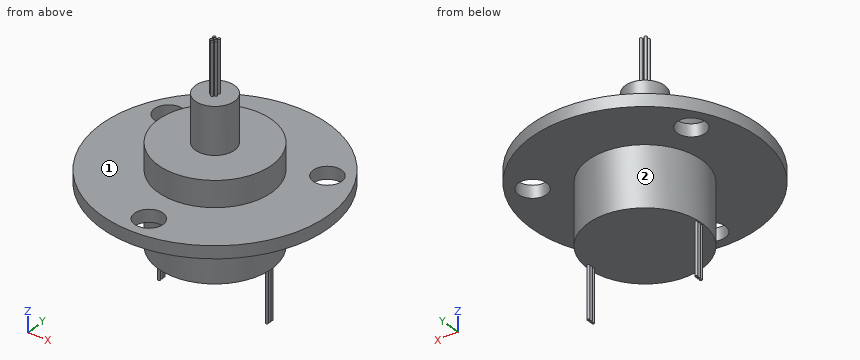
```python
from build123d import *

# Parameters (mm, degrees)
SKETCH1_W                      = 22
SKETCH1_H                      = 2.4
SKETCH2_R                      = 11
BOSS_EXTRUDE1_DEPTH            = 5
SKETCH3_R                      = 3.8
BOSS_EXTRUDE2_DEPTH            = 9
SKETCH4_R                      = 0.25
BOSS_EXTRUDE3_DEPTH            = 10
SKETCH5_R                      = 11
BOSS_EXTRUDE4_DEPTH            = 11.6
SKETCH6_W                      = 0.25
SKETCH6_H                      = 10
SKETCH7_W                      = 0.25
SKETCH7_H                      = 10
SKETCH8_W                      = 0.25
SKETCH8_H                      = 10
SKETCH9_W                      = 0.25
SKETCH9_H                      = 10
SKETCH10_W                     = 0.25
SKETCH10_H                     = 10
SKETCH11_W                     = 0.25
SKETCH11_H                     = 10
SKETCH12_W                     = 0.25
SKETCH12_H                     = 10
SKETCH13_W                     = 0.25
SKETCH13_H                     = 10
SKETCH14_W                     = 0.25
SKETCH14_H                     = 10
SKETCH15_W                     = 0.25
SKETCH15_H                     = 10
SKETCH16_W                     = 0.25
SKETCH16_H                     = 10
F_5_5_5_5_DIAMETER_HOLE1_D     = 5.5
F_5_5_5_5_DIAMETER_HOLE1_DEPTH = 26.4


with BuildPart() as part:
    # Sketch1 → Revolve1 (revolve)
    with BuildSketch(Plane.XZ):
        with Locations((11, 1.2)):
            Rectangle(SKETCH1_W, SKETCH1_H)
    revolve(axis=Axis((0, 0, 2.4), (0, 0, -1)))

    # Sketch2 → Boss-Extrude1 (add)
    with BuildSketch(Plane.XY.offset(2.4)):
        Circle(SKETCH2_R)
    extrude(amount=BOSS_EXTRUDE1_DEPTH)

    # Sketch3 → Boss-Extrude2 (add)
    with BuildSketch(Plane.XY.offset(7.4)):
        Circle(SKETCH3_R)
    extrude(amount=BOSS_EXTRUDE2_DEPTH)

    # Sketch4 → Boss-Extrude3 (add)
    with BuildSketch(Plane.XY.offset(16.4)):
        Circle(SKETCH4_R)
    extrude(amount=BOSS_EXTRUDE3_DEPTH)

    # Sketch5 → Boss-Extrude4 (add)
    with BuildSketch(Plane(origin=(0, 0, 0), x_dir=(-1, 0, 0), z_dir=(0, 0, -1))):
        Circle(SKETCH5_R)
    extrude(amount=BOSS_EXTRUDE4_DEPTH)

    # Sketch6 → Revolve2 (revolve)
    with BuildSketch(Plane.XZ.offset(0.816347149)):
        with Locations((0.163253006, 21.4)):
            Rectangle(SKETCH6_W, SKETCH6_H)
    revolve(axis=Axis((0.038253006, -0.816347149, 26.4), (0, 0, -1)))

    # Sketch7 → Revolve3 (revolve)
    with BuildSketch(Plane.XZ.offset(0.416347149)):
        with Locations((0.613253006, 21.4)):
            Rectangle(SKETCH7_W, SKETCH7_H)
    revolve(axis=Axis((0.488253006, -0.416347149, 26.4), (0, 0, -1)))

    # Sketch8 → Revolve4 (revolve)
    with BuildSketch(Plane.XZ.offset(-0.383652851)):
        with Locations((-0.286746994, 21.4)):
            Rectangle(SKETCH8_W, SKETCH8_H)
    revolve(axis=Axis((-0.411746994, 0.383652851, 26.4), (0, 0, -1)))

    # Sketch9 → Revolve5 (revolve)
    with BuildSketch(Plane.XZ.offset(-0.400094572)):
        with Locations((0.572352369, 21.4)):
            Rectangle(SKETCH9_W, SKETCH9_H)
    revolve(axis=Axis((0.447352369, 0.400094572, 26.4), (0, 0, -1)))

    # Sketch10 → Revolve6 (revolve)
    with BuildSketch(Plane(origin=(0, -0.222432877, 0), x_dir=(1, 0, 0), z_dir=(0, 1, 0))):
        with Locations((-10.392433295, 16.6)):
            Rectangle(SKETCH10_W, SKETCH10_H)
    revolve(axis=Axis((-10.517433295, -0.222432877, -21.6), (0, 0, 1)))

    # Sketch11 → Revolve7 (revolve)
    with BuildSketch(Plane(origin=(0, 0.377567123, 0), x_dir=(1, 0, 0), z_dir=(0, 1, 0))):
        with Locations((-10.392433295, 16.6)):
            Rectangle(SKETCH11_W, SKETCH11_H)
    revolve(axis=Axis((-10.517433295, 0.377567123, -21.6), (0, 0, 1)))

    # Sketch12 → Revolve8 (revolve)
    with BuildSketch(Plane(origin=(0, 0.6, 0), x_dir=(1, 0, 0), z_dir=(0, 1, 0))):
        with Locations((10.496693215, 16.6)):
            Rectangle(SKETCH12_W, SKETCH12_H)
    revolve(axis=Axis((10.371693215, 0.6, -21.6), (0, 0, 1)))

    # Sketch13 → Revolve9 (revolve)
    with BuildSketch(Plane(origin=(0, 0, 0), x_dir=(1, 0, 0), z_dir=(0, 1, 0))):
        with Locations((10.496693215, 16.6)):
            Rectangle(SKETCH13_W, SKETCH13_H)
    revolve(axis=Axis((10.371693215, 0, -21.6), (0, 0, 1)))

    # Sketch14 → Revolve10 (revolve)
    with BuildSketch(Plane(origin=(0, -0.6, 0), x_dir=(1, 0, 0), z_dir=(0, 1, 0))):
        with Locations((10.496693215, 16.6)):
            Rectangle(SKETCH14_W, SKETCH14_H)
    revolve(axis=Axis((10.371693215, -0.6, -21.6), (0, 0, 1)))

    # Sketch15 → Revolve11 (revolve)
    with BuildSketch(Plane(origin=(0, 0.968647222, 0), x_dir=(1, 0, 0), z_dir=(0, 1, 0))):
        with Locations((-10.392433295, 16.6)):
            Rectangle(SKETCH15_W, SKETCH15_H)
    revolve(axis=Axis((-10.517433295, 0.968647222, -21.6), (0, 0, 1)))

    # Sketch16 → Revolve12 (revolve)
    with BuildSketch(Plane.XZ.offset(0.416347149)):
        with Locations((-0.286746994, 21.4)):
            Rectangle(SKETCH16_W, SKETCH16_H)
    revolve(axis=Axis((-0.411746994, -0.416347149, 26.4), (0, 0, -1)))

    # Ø5.5 (5.5) Diameter Hole1
    with Locations(Plane(origin=(0, 0, 0), x_dir=(-1, 0, 0), z_dir=(0, 0, -1))):
        with Locations((-15.155444566, 8.75), (15.155444566, 8.75), (0, -17.5)):
            Hole(F_5_5_5_5_DIAMETER_HOLE1_D / 2, depth=F_5_5_5_5_DIAMETER_HOLE1_DEPTH)


solid = part.part
```
Model file for the job. Use its own axes, mm. Face numbers are marked on the shaded views. A direction names the side the tool comes from. Coordinates: 2 decimals unless noted, no trailing zeros. Order: outer loops, then holes, each group sorted by start corner. A loop starts at its lowest first (then second) coordinate and runs counter-clockwise, first axis right, second up. Notation, with made-up numbers: M 54,19.25 L 82,19.25 A31 cw 82,46.25 Z; hole C 46,-26 d9. An arc over 180 degrees is marked long. Answer as CSV lines item,"result".
(1) Band-saw the part on A-A, the plane x = -2. List the corners of the cut face in (y, z), then the cut area to 3 significant figures.
Geometry says:
outline,"M -21.91,0 L -19.39,0 L -19.39,2.4 L -21.91,2.4 Z; M -15.61,0 L -10.82,0 L -10.82,-11.6 L 10.82,-11.6 L 10.82,0 L 21.91,0 L 21.91,2.4 L 10.82,2.4 L 10.82,7.4 L 3.23,7.4 L 3.23,16.4 L -3.23,16.4 L -3.23,7.4 L -10.82,7.4 L -10.82,2.4 L -15.61,2.4 Z"
area,"513 mm2"
(2) Wall check: line 1 along X through (y, z) = (8, 1); line 2 along Y through (x, z) = (-0.5, 16.5); line 3 along Z through (x, y) = (-5, -11). Give the ranges that are in metal, low to high.
Geometry says:
line 1,"x = -20.49 to -17.8, -12.51 to 12.51, 17.8 to 20.49"
line 2,"y = -0.65 to -0.18, 0.15 to 0.62"
line 3,"z = 0 to 2.4"
(3) Band-saw the part on D-D, the plane y = -9.5. List the corners of the cut face in (x, z).
Geometry says:
outline,"M -19.84,0 L -5.55,0 L -5.55,-11.6 L 5.55,-11.6 L 5.55,0 L 19.84,0 L 19.84,2.4 L 5.55,2.4 L 5.55,7.4 L -5.55,7.4 L -5.55,2.4 L -19.84,2.4 Z"
(4) 3-axis set-ups, long thin cutter, end or side, ignore diameter. For the marked faces 1 and 2: which of +Z, -Z, +X, -X, +Y, -Y reach the whole face in a straight line?
Geometry says:
face 1,"+Z"
face 2,"-Z"
(5) Band-saw the part on C-C, the plane z = 17.5. List the corners of the cut face in (x, y).
Geometry says:
outline,"C -0.41,-0.42 d0.5; C -0.41,0.38 d0.5; C 0,0 d0.5; C 0.04,-0.82 d0.5; C 0.45,0.4 d0.5; C 0.49,-0.42 d0.5"
(6) Flat gauge pins, fed straight in: pin 1 (10 mm diameter, centred on x = -1, z = 20, fed in from -Y); pin 2 (3 mm diameter, centred on x = -8, z = -12.5, fed in from +Y); pin 3 (6.5 mm diameter, centred on x = 15.16, y = 8.75, fed in from +Z). Where does each tip first touch, or does it go through?
Geometry says:
pin 1,"stops at y = -3.8"
pin 2,"stops at y = 8.65"
pin 3,"stops at z = 2.4"
(7) Band-saw the part on B-B, the plane y = -17.5. List the corners of the cut face in (x, z).
Geometry says:
outline,"M -13.33,0 L -2.75,0 L -2.75,2.4 L -13.33,2.4 Z; M 2.75,0 L 13.33,0 L 13.33,2.4 L 2.75,2.4 Z"
